from build123d import *

# Parameters (mm, degrees)
SKETCH_1_W          = 10
SKETCH_1_H          = 20
SKETCH_1_W_2        = 7.6
SKETCH_1_H_2        = 17.6
EXTRUDE_1_DEPTH     = 665
SKETCH_2_R          = 2
CUT_EXTRUDE_1_DEPTH = 666.150358941
SKETCH_3_R          = 2
CUT_EXTRUDE_2_DEPTH = 666.319472134


with BuildPart() as part:
    # ｽｹｯﾁ1 → 押し出し-薄板1 (new body)
    with BuildSketch(Plane(origin=(0, 0, 0), x_dir=(0, 0, -1), z_dir=(1, 0, 0))):
        Rectangle(SKETCH_1_W, SKETCH_1_H)
        Rectangle(SKETCH_1_W_2, SKETCH_1_H_2, mode=Mode.SUBTRACT)
    extrude(amount=EXTRUDE_1_DEPTH)

    # ｽｹｯﾁ2 → ｶｯﾄ - 押し出し1 (cut, through all)
    with BuildSketch(Plane.XY.offset(5)):
        with Locations((25, 0)):
            Circle(SKETCH_2_R)
        with Locations(Location((640, 0, 0), (0, 0, 90))):
            Circle(SKETCH_2_R)
        with Locations((50, 0)):
            Circle(SKETCH_2_R)
        with Locations(Location((615, 0, 0), (0, 0, 90))):
            Circle(SKETCH_2_R)
        with Locations((320, 5)):
            Circle(SKETCH_2_R)
        with Locations((320, -5)):
            Circle(SKETCH_2_R)
        with Locations(Location((345, -5, 0), (0, 0, 90))):
            Circle(SKETCH_2_R)
        with Locations(Location((345, 5, 0), (0, 0, 90))):
            Circle(SKETCH_2_R)
        with Locations((332.5, 5)):
            Circle(SKETCH_2_R)
        with Locations(Location((332.5, -5, 0), (0, 0, 90))):
            Circle(SKETCH_2_R)
    extrude(amount=-CUT_EXTRUDE_1_DEPTH, mode=Mode.SUBTRACT)

    # ｽｹｯﾁ3 → ｶｯﾄ - 押し出し2 (cut, through all)
    with BuildSketch(Plane(origin=(0, 10, 0), x_dir=(1, 0, 0), z_dir=(0, 1, 0))):
        with Locations(Location((5, 0, 0), (0, 0, 270))):
            Circle(SKETCH_3_R)
        with Locations(Location((130, 0, 0), (0, 0, 270))):
            Circle(SKETCH_3_R)
        with Locations(Location((535, 0, 0), (0, 0, 270))):
            Circle(SKETCH_3_R)
        with Locations(Location((660, 0, 0), (0, 0, 270))):
            Circle(SKETCH_3_R)
        with Locations(Location((25, 0, 0), (0, 0, 270))):
            Circle(SKETCH_3_R)
        with Locations(Location((640, 0, 0), (0, 0, 270))):
            Circle(SKETCH_3_R)
    extrude(amount=-CUT_EXTRUDE_2_DEPTH, mode=Mode.SUBTRACT)


solid = part.part
Geometry check sheet. Reference: the model listing, model coordinates, mm. A direction names the side the tool comes from. Give positions to 0.01 mm unless a question says otherwise; leave off trailing zeros. Loops run counter-clockwise (first coordinate to the right, second up) from the corner with the lowest first, then second, coordinate; pieces in that order, holes last. Notation, with made-up numbers: (34.25, 31.25) -> (60.25, 31.25) arc R28 ccw to (60.25, 64.25) -> close; hole circle Ø10 at (-3, -22.5). An arc over 180 degrees is marked (long way). Answer in a Markdown table with one row per item. Add a question column.
1) Cross-section at A-A on x = 140.5. Record the boundary of the cut face in (y, z).
2) Set-up check for faces 1 (the face through (328, 0, -3.8)), 2 (the face through (328, 0, -5)): record each of +Z, -Z, +X, -X, +Y, -Y from which the full face is reachable in a straight line by a thin tool's end or side.
3) Cross-section at B-B on z = 0.25. State how many separate pieces and enclosed holes the cut face has, and give its area (3 significant figures).
4) Draft check along Y on faces 3 (the face through (328, 0, 3.8)), 4 (the face through (328, 0, 5)), 5 (the face through (328, -10, 0)). Enter one of: pulls with the +Y half, pulls with the -Y half, needs draft (parallel to the pull), parting line crosses it, or undercut.
5) Material ranges on probe 1 along Y at (x, z) = (332.5, -4.15); probe 2 along Z at (x, y) = (236.5, 2.5); probe 3 along Y at (x, z) = (25, 4.8), recorded low to high. Write a range as from..to.
Outcome:
| question | item | result |
|---|---|---|
| 1 | outline | (-10, -5) -> (10, -5) -> (10, 5) -> (-10, 5) -> close; hole (-8.8, -3.8) -> (8.8, -3.8) -> (8.8, 3.8) -> (-8.8, 3.8) -> close |
| 2 | face 1 | +X, -X |
| 2 | face 2 | -Z, +X, -X, +Y, -Y |
| 3 | separate pieces | 14 |
| 3 | enclosed holes | 0 |
| 3 | area | 1,540 mm^2 |
| 4 | face 3 | undercut |
| 4 | face 4 | needs draft |
| 4 | face 5 | pulls with the -Y half |
| 5 | probe 1 | y = -10..-7, -3..3, 7..10 |
| 5 | probe 2 | z = -5..-3.8, 3.8..5 |
| 5 | probe 3 | y = -10..-2, 2..10 |
